```python
from build123d import *

# Parameters (mm, degrees)
BASE_FLANGE1_DEPTH              = 1.2192
HOLE1_START                     = -1.2192
HOLE1_OUTLINE_R                 = 1.0922
HOLE1_DEPTH                     = 1.2192
EDGE_FLANGE1_DEPTH              = 6.35
F_1_CLEARANCE_HOLE2_D           = 2.0574
F_1_CLEARANCE_HOLE2_ON_FACE_2_D = 2.0574
F_2_CLEARANCE_HOLE2_D           = 2.4384


# Read off the part's stored shape, not the designer's step: Hole1
# Sheet-metal steps are written as plain solids
with BuildPart() as part:
    # Sketch1 → Base-Flange1 (new body)
    with BuildSketch(Plane(origin=(0, 0, 0), x_dir=(1, 0, 0), z_dir=(0, 1, 0))):
        with BuildLine():
            Line((4.02700332, 6.35), (15.890507526, 9.528816371))
            Line((15.890507526, 9.528816371), (17.534008462, 3.395187374))
            Line((17.534008462, 3.395187374), (5.266750468, 0.108185502))
            ThreePointArc((5.266750468, 0.108185502), (4.939943157, 0.001343981), (4.626605284, -0.140209919))
            Line((4.626605284, -0.140209919), (0, -2.54))
            Line((0, -2.54), (-3.81, -2.54))
            Line((-3.81, -2.54), (-3.81, 6.35))
            Line((-3.81, 6.35), (4.02700332, 6.35))
        make_face()
    extrude(amount=-BASE_FLANGE1_DEPTH)

    # Hole1 outline → Hole1 (cut)
    with BuildSketch(Plane(origin=(0, 0, 0), x_dir=(1, 0, 0), z_dir=(0, 1, 0)).offset(HOLE1_START)):
        with Locations((4.445, 3.175)):
            Circle(HOLE1_OUTLINE_R)
    extrude(amount=HOLE1_DEPTH, mode=Mode.SUBTRACT)

    # Edge-Flange1 section (across the edge) → Edge-Flange1 (add)
    with BuildSketch(Plane(origin=(18.388628949, -1.2192, -0.205700296), x_dir=(-0.2588190451025216, -3.4914813388431334e-15, -0.9659258262890682), z_dir=(-0.9659258262890682, 0, 0.2588190451025216))):
        with BuildLine():
            Line((-1.2192, 0.762), (-1.2192, 12.7))
            Line((-1.2192, 12.7), (0, 12.7))
            Line((0, 12.7), (0, 0.762))
            ThreePointArc((0, 0.762), (0.223184633, 0.223184633), (0.762, 0))
            Line((0.762, 0), (3.302, 0))
            Line((3.302, 0), (3.302, -1.2192))
            Line((3.302, -1.2192), (0.762, -1.2192))
            ThreePointArc((0.762, -1.2192), (-0.638919955, -0.638919955), (-1.2192, 0.762))
        make_face()
    extrude(amount=EDGE_FLANGE1_DEPTH)

    # #1 Clearance Hole2 (through all)
    with Locations(Plane(origin=(17.16190315, -10.4902, 0.122999891), x_dir=(-0.965925826289, 0, 0.258819045103), z_dir=(-0.258819045103, 0, -0.965925826289))):
        with Locations((0, 0)):
            Hole(F_1_CLEARANCE_HOLE2_D / 2)

    # #1 Clearance Hole2 on face 2 (through all)
    with Locations(Plane(origin=(17.16190315, -5.4102, 0.122999891), x_dir=(-0.965925849201, 0, 0.258818959594), z_dir=(-0.258818959594, 0, -0.965925849201))):
        with Locations((0, 0)):
            Hole(F_1_CLEARANCE_HOLE2_ON_FACE_2_D / 2)

    # #2 Clearance Hole2 (through all)
    with Locations(Plane(origin=(0, 0, 0), x_dir=(1, 0, 0), z_dir=(0, 1, 0))):
        with Locations((-1.905, 0), (-1.905, 3.81)):
            Hole(F_2_CLEARANCE_HOLE2_D / 2)


solid = part.part
```
Verification items for the finished model (mm, model axes). A direction names the side the tool comes from. Coordinates: 2 decimals unless noted, no trailing zeros. Order: outer loops, then holes, each group sorted by start corner. A loop starts at its lowest first (then second) coordinate and runs counter-clockwise, first axis right, second up. Notation, with made-up numbers: (43.5, 12) - (89.5, 12) arc R34 cw to (89.5, 43) - close; hole circle Ø1 at (36, 20). An arc over 180 degrees is marked (long way). Return JSON: item names as keys, results as strings.
(1) Section check C-C, the plane y = -7.5. Record the cut outline in (x, z) (3 decimals), and give its area (3 significant figures).
Filled sheet:
{"outline": "(12.255, 1.438) - (18.389, -0.206) - (18.704, 0.972) - (12.571, 2.615) - close", "area": "7.74 mm^2"}
(2) Thickness scan on line 1 along Y through (x, z) = (10, -3); line 2 along Z through (x, y) = (14, -9.5); line 3 along Z through (x, y) = (13.25, -4.25). Record the ranges inside material, lowest first.
Filled sheet:
{"line 1": "y = -1.22 to 0", "line 2": "z = 0.97 to 2.23", "line 3": "z = 1.17 to 2.43"}
(3) Section check D-D, the plane x = 11.75. Record the cut outline in (y, z).
Filled sheet:
{"outline": "(-1.22, -8.42) - (0, -8.42) - (0, -0.45) - (-1.22, -0.45) - close"}
(4) Mould release check, pull along X, two halves, no side actions. Record for faces 4 (the cylindrical face through (17.106, -6.414, 0.778)), 5 (the cylindrical face through (15.526, -0.565, 1.207)), 6 (the flat face through (9.88, -0.6, -7.92)): pulls with the +X half, pulls with the -X half, needs draft (parallel to the pull), parting line crosses it, or undercut.
Filled sheet:
{"face 4": "undercut", "face 5": "pulls with the +X half", "face 6": "pulls with the -X half"}
(5) Go/stop test with flat-tipped pins: pin 1 (5 mm diameter, centred on x = 7.5, y = -3.5, fed in from -Z); pin 2 (8 mm diameter, centred on x = 10.5, y = -7, fed in from +Z); pin 3 (3 mm diameter, centred on x = -1.905, z = 0, fed in from -Y). Record where each tip stops, or that it passes through.
Filled sheet:
{"pin 1": "stops at z = -7.55", "pin 2": "stops at z = 2.62", "pin 3": "stops at y = -1.22"}
(6) Section check A-A, the plane y = -10.75. Record the cut outline in (x, z) (3 decimals).
Filled sheet:
{"outline": "(12.255, 1.438) - (16.2, 0.381) - (16.516, 1.558) - (12.571, 2.615) - close; (18.123, -0.135) - (18.389, -0.206) - (18.704, 0.972) - (18.439, 1.043) - close"}
(7) Section check B-B, the plane z = -3.81. Record the cut outline in (x, y).
Filled sheet:
{"outline": "(-3.81, -1.22) - (-3.12, -1.22) - (-3.12, 0) - (-3.81, 0) - close; (-0.69, -1.22) - (3.56, -1.22) - (3.56, 0) - (-0.69, 0) - close; (5.33, -1.22) - (17.42, -1.22) - (17.42, 0) - (5.33, 0) - close"}
(8) Access from +Z, -Z, +X, -X, +Y, -Y to the whole of each face (thin tool, end or side, straight path). Record for faces 1 (the flat face through (15.365, -8.034, 0.605)), 2 (the flat face through (2.35, -0.6, 1.32)), 3 (the flat face through (0, -1, -6.35)).
Filled sheet:
{"face 1": "-Z, -X, -Y", "face 2": "+Z, +Y, -Y", "face 3": "-Z, -X, +Y, -Y"}
